from build123d import *

# Parameters (mm, degrees)
SKETCH2_R               = 104.775
SKETCH2_R_2             = 98.425
BOSS_EXTRUDE1_DEPTH     = 304.8
SKETCH3_R               = 130.175
SKETCH3_R_2             = 104.775
BOSS_EXTRUDE3_DEPTH     = 6.35
F_1_2_CLEARANCE_HOLE1_D = 13.49248
CIRPATTERN1_COUNT       = 12
MIRROR2_COPY_1_D        = 13.49248
MIRROR2_COPY_2_D        = 13.49248
MIRROR2_COPY_3_D        = 13.49248
MIRROR2_COPY_4_D        = 13.49248
MIRROR2_COPY_5_D        = 13.49248
MIRROR2_COPY_6_D        = 13.49248
MIRROR2_COPY_7_D        = 13.49248
MIRROR2_COPY_8_D        = 13.49248
MIRROR2_COPY_9_D        = 13.49248
MIRROR2_COPY_10_D       = 13.49248
MIRROR2_COPY_11_D       = 13.49248


with BuildPart() as part:
    # Sketch2 → Boss-Extrude1 (new body)
    with BuildSketch(Plane.XY):
        with Locations(Location((0, 0, 0), (0, 0, 180))):
            Circle(SKETCH2_R)
        with Locations(Location((0, 0, 0), (0, 0, 180))):
            Circle(SKETCH2_R_2, mode=Mode.SUBTRACT)
    boss_extrude1 = extrude(amount=BOSS_EXTRUDE1_DEPTH)

    # Sketch3 → Boss-Extrude3 (add)
    with BuildSketch(Plane(origin=(0, 0, 0), x_dir=(-1, 0, 0), z_dir=(0, 0, -1))):
        Circle(SKETCH3_R)
        Circle(SKETCH3_R_2, mode=Mode.SUBTRACT)
    boss_extrude3 = extrude(amount=-BOSS_EXTRUDE3_DEPTH)

    # 1/2 Clearance Hole1 (through all)
    with Locations(Plane(origin=(0, 0, 0), x_dir=(-1, 0, 0), z_dir=(0, 0, -1))):
        with Locations((0, 117.475)):
            f_1_2_clearance_hole1 = Hole(F_1_2_CLEARANCE_HOLE1_D / 2)

    # CirPattern1: 1/2 Clearance Hole1 ×12 about axis
    cirpattern1_axis = Axis((0, 0, 0), (0, 0, 1))
    for i in range(1, CIRPATTERN1_COUNT):
        add(f_1_2_clearance_hole1.rotate(cirpattern1_axis, i * 360 / CIRPATTERN1_COUNT), mode=Mode.SUBTRACT)

    # Mirror2: Boss-Extrude1, Boss-Extrude3, 1/2 Clearance Hole1 across plane
    add(boss_extrude1.mirror(Plane.XY.offset(155.575)))
    add(boss_extrude3.mirror(Plane.XY.offset(155.575)))
    add(f_1_2_clearance_hole1.mirror(Plane.XY.offset(155.575)), mode=Mode.SUBTRACT)

    # Mirror2 copy 1 (through all)
    with Locations(Plane(origin=(0, 0, 311.15), x_dir=(-0.8660254037844387, -0.49999999999999994, 0), z_dir=(0, 0, 1))):
        with Locations((0, -117.475)):
            Hole(MIRROR2_COPY_1_D / 2)

    # Mirror2 copy 2 (through all)
    with Locations(Plane(origin=(0, 0, 311.15), x_dir=(-0.5000000000000001, -0.8660254037844386, 0), z_dir=(0, 0, 1))):
        with Locations((0, -117.475)):
            Hole(MIRROR2_COPY_2_D / 2)

    # Mirror2 copy 3 (through all)
    with Locations(Plane(origin=(0, 0, 311.15), x_dir=(0, -1, 0), z_dir=(0, 0, 1))):
        with Locations((0, -117.475)):
            Hole(MIRROR2_COPY_3_D / 2)

    # Mirror2 copy 4 (through all)
    with Locations(Plane(origin=(0, 0, 311.15), x_dir=(0.4999999999999998, -0.8660254037844387, 0), z_dir=(0, 0, 1))):
        with Locations((0, -117.475)):
            Hole(MIRROR2_COPY_4_D / 2)

    # Mirror2 copy 5 (through all)
    with Locations(Plane(origin=(0, 0, 311.15), x_dir=(0.8660254037844387, -0.49999999999999994, 0), z_dir=(0, 0, 1))):
        with Locations((0, -117.475)):
            Hole(MIRROR2_COPY_5_D / 2)

    # Mirror2 copy 6 (through all)
    with Locations(Plane.XY.offset(311.15)):
        with Locations((0, -117.475)):
            Hole(MIRROR2_COPY_6_D / 2)

    # Mirror2 copy 7 (through all)
    with Locations(Plane(origin=(0, 0, 311.15), x_dir=(0.8660254037844386, 0.5000000000000001, 0), z_dir=(0, 0, 1))):
        with Locations((0, -117.475)):
            Hole(MIRROR2_COPY_7_D / 2)

    # Mirror2 copy 8 (through all)
    with Locations(Plane(origin=(0, 0, 311.15), x_dir=(0.5000000000000004, 0.8660254037844384, 0), z_dir=(0, 0, 1))):
        with Locations((0, -117.475)):
            Hole(MIRROR2_COPY_8_D / 2)

    # Mirror2 copy 9 (through all)
    with Locations(Plane(origin=(0, 0, 311.15), x_dir=(0, 1, 0), z_dir=(0, 0, 1))):
        with Locations((0, -117.475)):
            Hole(MIRROR2_COPY_9_D / 2)

    # Mirror2 copy 10 (through all)
    with Locations(Plane(origin=(0, 0, 311.15), x_dir=(-0.5000000000000001, 0.8660254037844386, 0), z_dir=(0, 0, 1))):
        with Locations((0, -117.475)):
            Hole(MIRROR2_COPY_10_D / 2)

    # Mirror2 copy 11 (through all)
    with Locations(Plane(origin=(0, 0, 311.15), x_dir=(-0.8660254037844384, 0.5000000000000004, 0), z_dir=(0, 0, 1))):
        with Locations((0, -117.475)):
            Hole(MIRROR2_COPY_11_D / 2)


solid = part.part
Read the model definition and answer for the solid it produces. Units are mm, in the model's axes. A direction names the side the tool comes from. Round coordinates to 2 decimals unless told otherwise and drop trailing zeros. Write each loop counter-clockwise with the first axis right and the second up, starting at its lowest first coordinate (ties: lowest second). Pieces come first, ordered by that corner, then holes.
Q1. Find section D-D on x = -43. Determine the outline of the cut face in (y, z).
Values:
outline: (-122.87, 0) - (-88.54, 0) - (-88.54, 311.15) - (-122.87, 311.15) - (-122.87, 304.8) - (-95.54, 304.8) - (-95.54, 6.35) - (-122.87, 6.35) - close; (88.54, 0) - (122.87, 0) - (122.87, 6.35) - (95.54, 6.35) - (95.54, 304.8) - (122.87, 304.8) - (122.87, 311.15) - (88.54, 311.15) - close
Q2. The mould has two halves that part along Y. Classify faces 3 (the face through (-96.38, 62.84, 3.22)), 4 (the face through (87.4, 58.5, 6.35)), 5 (the face through (22.713, 102.283, 157.664)): released by +Y, released by -Y, zero draft, split by the parting line, or undercut.
Values:
face 3: undercut
face 4: zero draft
face 5: split by the parting line
Q3. Find section C-C on z = 188. Determine the outline of the cut face in (x, y) (3 decimals), and give its area (3 significant figures).
Values:
outline: circle Ø209.55 at (0, 0); hole circle Ø196.85 at (0, 0)
area: 4,050 mm2
Q4. Flat-ended cylindrical pins translate along their axes: P1, Ø15.5, axis at x = 101.74, y = -58.74, coming from the -Z side; P2, Ø6, axis at x = -82.5, z = 109, coming from the +Y side; P3, Ø6, axis at x = -36.5, z = 40, coming from the -Y side; P4, Ø5, axis at x = 46.5, z = 182.5, coming from the -Y side. Find the tip coordinate at first contact, or state that the pin passes through.
Values:
P1: stops at z = 0
P2: stops at y = 68.25
P3: stops at y = -99.28
P4: stops at y = -95.09
Q5. A tool of negligible diameter and unlimited length cuts with its end or side. For faces 1 (the face through (87.4, 58.5, 304.8)), 2 (the face through (56.71, -95.3, 3.22)), from which of +Z, -Z, +X, -X, +Y, -Y can it reach the whole face along a straight path? Write none if from no direction.
Values:
face 1: none
face 2: +Z, -Z
Q6. Find section A-A on y = 0. State how many separate pieces and enclosed holes the cut face has, and give its area (3 significant figures).
Values:
separate pieces: 6
enclosed holes: 0
area: 4,250 mm2
Q7. Straight lines are drawn through the part: line 1 (Y direction, x = 0, z = 308.75) (3 decimals); line 2 (Y direction, x = 2, z = 117). For each, find the intervals that lie inside material, in ascending order.
Values:
line 1: y = -130.175 to -124.221, -110.729 to -98.425, 98.425 to 110.729, 124.221 to 130.175
line 2: y = -104.76 to -98.4, 98.4 to 104.76
